Could you check a few things on this model? Use its own coordinates, in mm. Face numbers are marked on the shaded views. A direction names the side the tool comes from. Round coordinates to 2 decimals unless told otherwise and drop trailing zeros. Loops run counter-clockwise (first coordinate to the right, second up) from the corner with the lowest first, then second, coordinate; pieces in that order, holes last. Notation, with made-up numbers: (52.25, 15.5) - (89.25, 15.5) arc R20 cw to (89.25, 28.5) - close; hole circle Ø2 at (70, -39.75). An arc over 180 degrees is marked (long way). Use one line per item in the form item = value.
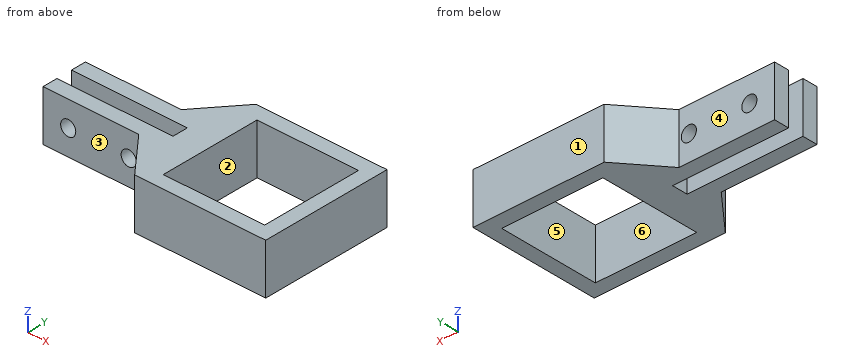
```python
from build123d import *

# Parameters (mm, degrees)
EXTRUDE_1_DEPTH     = 10
SKETCH_5_W          = 20.1
SKETCH_5_H          = 20.1
CUT_EXTRUDE_1_DEPTH = 30
SKETCH_7_R          = 1.5
CUT_EXTRUDE_5_DEPTH = 9.1


with BuildPart() as part:
    # 草图1 → 凸台-拉伸1 (new body)
    with BuildSketch(Plane.XY):
        Polygon((-26, 4.55), (-26, 1.55), (-3, 1.55), (-3, -1.55), (-26, -1.55), (-26, -4.55), (-7, -4.55), (0, -13), (26, -13), (26, 13), (0, 13), (-7, 4.55), align=None)
    extrude(amount=EXTRUDE_1_DEPTH)

    # 草图5 → 切除-拉伸1 (cut)
    with BuildSketch(Plane.XY.offset(10)):
        with Locations((13.05, -0.05)):
            Rectangle(SKETCH_5_W, SKETCH_5_H)
    extrude(amount=-CUT_EXTRUDE_1_DEPTH, mode=Mode.SUBTRACT)

    # 草图7 → 切除-拉伸5 (cut)
    with BuildSketch(Plane(origin=(0, 4.55, 0), x_dir=(1, 0, 0), z_dir=(0, 1, 0))):
        with Locations((-21, -5)):
            Circle(SKETCH_7_R)
        with Locations((-9, -5)):
            Circle(SKETCH_7_R)
    extrude(amount=-CUT_EXTRUDE_5_DEPTH, mode=Mode.SUBTRACT)


solid = part.part
```
1. On a 3-axis mill with a long thin cutter (end or side, diameter ignored), from which of +Z, -Z, +X, -X, +Y, -Y can I reach the whole of each face in a straight line? I mean the marked faces 1 and 2. Say none if no direction works.
Solution:
face_1 = +Z, -Z, +X, -X, +Y
face_2 = +Z, -Z
2. If we section it at C-C, the plane z = 8.75: Write out the boundary of the cut face in (x, y).
Solution:
outline = (-26, -4.55) - (-7, -4.55) - (0, -13) - (26, -13) - (26, 13) - (0, 13) - (-7, 4.55) - (-26, 4.55) - (-26, 1.55) - (-3, 1.55) - (-3, -1.55) - (-26, -1.55) - close; hole (3, -10.1) - (23.1, -10.1) - (23.1, 10) - (3, 10) - close
3. Please list where these lines run through material, in increasing order: line 1 along X through (y, z) = (2.6, 5); line 2 along Z through (x, y) = (-21, 2.75); line 3 along Y through (x, z) = (7.5, 5.75).
Solution:
line_1 = -26 to -22.5, -19.5 to -10.5, -7.5 to 3, 23.1 to 26
line_2 = 0 to 3.5, 6.5 to 10
line_3 = -13 to -10.1, 10 to 13
4. If we section it at A-A, the plane x = -9: Write out the boundary of the cut face in (y, z).
Solution:
outline = (-4.55, 0) - (-1.55, 0) - (-1.55, 3.5) - (-4.55, 3.5) - close; (-4.55, 6.5) - (-1.55, 6.5) - (-1.55, 10) - (-4.55, 10) - close; (1.55, 0) - (4.55, 0) - (4.55, 3.5) - (1.55, 3.5) - close; (1.55, 6.5) - (4.55, 6.5) - (4.55, 10) - (1.55, 10) - close
5. If we section it at D-D, the plane x = 9.5: Write out the boundary of the cut face in (y, z), plus the area to 3 significant figures.
Solution:
outline = (-13, 0) - (-10.1, 0) - (-10.1, 10) - (-13, 10) - close; (10, 0) - (13, 0) - (13, 10) - (10, 10) - close
area = 59.0 mm^2
6. We'd pull the mould along Y, two halves only. Please class the marked faces 3, 4, 5 and 6: +Y half, -Y half, draft (parallel to the pull), parting line (faces both ways), or undercut.
Solution:
face_3 = -Y half
face_4 = +Y half
face_5 = undercut
face_6 = undercut
7. For P1, Ø5, axis at x = -16.5, z = 6, coming from the -Y side; P2, Ø1.8, axis at x = -9, z = 5, coming from the -Y side; P3, Ø5, axis at x = -9, z = 5, coming from the -Y side; P4, Ø2.5, axis at y = 0, z = 3.5, coming from the -X side, each with a flat end and sliding along its axis, tell me the tip position at first contact or that it passes through.
Solution:
P1 = -4.55
P2 = through
P3 = -5.15
P4 = -3
8. If we section it at B-B, the plane z = 5: Count the separate pieces of the cut face and the enclosed holes in it, plus the area to 3 significant figures.
Solution:
separate_pieces = 5
enclosed_holes = 1
area = 460 mm^2
